Geometry check sheet. Reference: the model listing, model coordinates, mm. Face numbers are marked on the shaded views. A direction names the side the tool comes from. Give positions to 0.01 mm unless a question says otherwise; leave off trailing zeros. Loops run counter-clockwise (first coordinate to the right, second up) from the corner with the lowest first, then second, coordinate; pieces in that order, holes last. Notation, with made-up numbers: (31.25, -18.5) -> (45.25, -18.5) arc R20 cw to (45.25, -12.5) -> close; hole circle Ø4 at (37.5, 85). An arc over 180 degrees is marked (long way). One line per question, with ' | ' between items.
from build123d import *

# Parameters (mm, degrees)
SKETCH1_W      = 7.96
SKETCH1_H      = 7.96
EXTRUDE1_DEPTH = 6.3
EXTRUDE2_DEPTH = 8.96
SHELL1_T       = -1.55
EXTRUDE4_DEPTH = 4.86
SKETCH6_W      = 7.96
SKETCH6_H      = 7.96
SKETCH6_W_2    = 7.56
SKETCH6_H_2    = 7.56
EXTRUDE5_DEPTH = 0.2
FILLET1_R      = 0.05


with BuildPart() as part:
    # Sketch1 → Extrude1 (new body)
    with BuildSketch(Plane(origin=(0, 0, 0), x_dir=(1, 0, 0), z_dir=(0, 1, 0))):
        Rectangle(SKETCH1_W, SKETCH1_H)
    extrude(amount=EXTRUDE1_DEPTH)

    # Sketch2 → Extrude2 (cut, through all)
    with BuildSketch(Plane(origin=(3.98, 0, 0), x_dir=(0, 0, -1), z_dir=(1, 0, 0))):
        Polygon((-3.98, 2.2), (3.98, 6.3), (-3.98, 6.3), align=None)
    extrude(amount=-EXTRUDE2_DEPTH, mode=Mode.SUBTRACT)

    # Shell1
    shell1_openings = [part.faces().sort_by_distance(p)[0] for p in [
        (0, 0, 0),
    ]]
    offset(amount=SHELL1_T, openings=shell1_openings, kind=Kind.INTERSECTION)

    # Sketch5 → Extrude4 (cut)
    with BuildSketch(Plane(origin=(-2.43, 0, 0), x_dir=(0, 0, -1), z_dir=(1, 0, 0))):
        Polygon((-2.43, 0), (2.43, 0), (2.43, 3.915585189), (-2.43, 1.412318857), align=None)
    extrude(amount=EXTRUDE4_DEPTH, mode=Mode.SUBTRACT)

    # Sketch6 → Extrude5 (cut)
    with BuildSketch(Plane.XZ):
        Rectangle(SKETCH6_W, SKETCH6_H)
        Rectangle(SKETCH6_W_2, SKETCH6_H_2, mode=Mode.SUBTRACT)
    extrude(amount=-EXTRUDE5_DEPTH, mode=Mode.SUBTRACT)

    # Fillet1
    fillet1_edges = [part.edges().sort_by_distance(p)[0] for p in [
        (3.98, 1.2, 3.98),
        (-3.98, 1.2, 3.98),
        (0, 2.2, 3.98),
        (-3.98, 4.25, 0),
        (3.98, 4.25, 0),
        (2.43, 0.706159428, 2.43),
        (2.43, 0, 0),
        (0, 0, -2.43),
        (2.43, 1.957792594, -2.43),
        (-2.43, 1.957792594, -2.43),
        (-2.43, 0, 0),
        (-2.43, 0.706159428, 2.43),
        (0, 0, 2.43),
        (2.43, 2.663952023, 0),
        (0, 3.915585189, -2.43),
        (-2.43, 2.663952023, 0),
        (0, 1.412318857, 2.43),
        (-3.98, 0.2, 0),
        (0, 0.2, 3.98),
        (3.98, 0.2, 0),
        (0, 0.2, -3.98),
        (-3.78, 0.2, 0),
        (0, 0.2, -3.78),
        (3.78, 0.2, 0),
        (0, 0.2, 3.78),
        (-3.78, 0, 0),
        (-3.78, 0.1, 3.78),
        (0, 0, 3.78),
        (3.78, 0.1, 3.78),
        (3.78, 0, 0),
        (3.78, 0.1, -3.78),
        (0, 0, -3.78),
        (-3.78, 0.1, -3.78),
        (0, 6.3, -3.98),
        (-3.98, 3.25, -3.98),
        (3.98, 3.25, -3.98),
    ]]
    fillet(fillet1_edges, radius=FILLET1_R)


solid = part.part
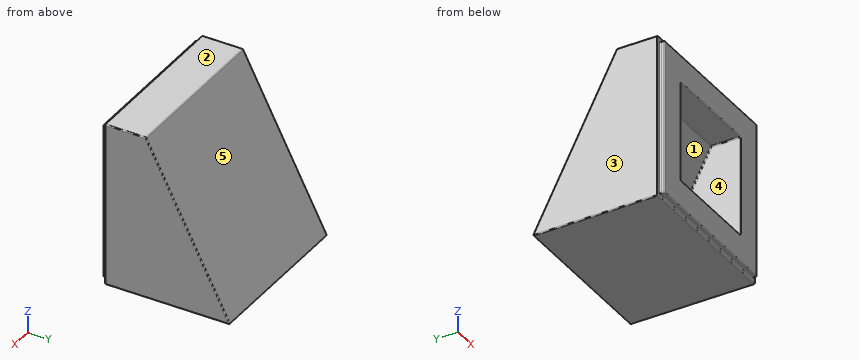
Item 1: Sectioned sample at B-B (x = -1.75). Record the cut outline in (y, z), plus the area to 3 significant figures.
Result:
outline: (0, -3.73) arc R0.05 ccw to (0.05, -3.78) -> (0.15, -3.78) arc R0.05 cw to (0.2, -3.83) -> (0.2, -3.93) arc R0.05 ccw to (0.25, -3.98) -> (6.22, -3.98) arc R0.05 ccw to (6.26, -3.91) -> (2.21, 3.95) arc R0.05 ccw to (2.17, 3.98) -> (0.25, 3.98) arc R0.05 ccw to (0.2, 3.93) -> (0.2, 3.83) arc R0.05 cw to (0.15, 3.78) -> (0.05, 3.78) arc R0.05 ccw to (0, 3.73) -> (0, 2.48) arc R0.05 ccw to (0.05, 2.43) -> (1.38, 2.43) arc R0.05 cw to (1.43, 2.4) -> (3.88, -2.36) arc R0.05 cw to (3.83, -2.43) -> (0.05, -2.43) arc R0.05 ccw to (0, -2.48) -> close | area: 20.8 mm2
Item 2: Sectioned sample at A-A (x = -3.25). Record the cut outline in (y, z), plus the area to 3 significant figures.
Result:
outline: (0, -3.73) arc R0.05 ccw to (0.05, -3.78) -> (0.15, -3.78) arc R0.05 cw to (0.2, -3.83) -> (0.2, -3.93) arc R0.05 ccw to (0.25, -3.98) -> (6.22, -3.98) arc R0.05 ccw to (6.26, -3.91) -> (2.21, 3.95) arc R0.05 ccw to (2.17, 3.98) -> (0.25, 3.98) arc R0.05 ccw to (0.2, 3.93) -> (0.2, 3.83) arc R0.05 cw to (0.15, 3.78) -> (0.05, 3.78) arc R0.05 ccw to (0, 3.73) -> close | area: 33.7 mm2
Item 3: Depth check by flat-ended pin: pin 1 Ø4 at (x, z) = (-0.5, 2) entering from +Y; pin 2 Ø2 at (x, z) = (-1.5, -2.5) entering from +Y. Enter the tip coordinate at first touch or a pass-through.
Result:
pin 1: y = 4.25 | pin 2: y = 6.05
Item 4: Scan lines: probe 1 along X at (y, z) = (0.5, 1); probe 2 along Z at (x, y) = (1, 5.5). Record each from-to range of solid material in increasing order.
Result:
probe 1: -3.98 to -2.43, 2.43 to 3.98 | probe 2: -3.98 to -2.43
Item 5: Set-up check for the marked faces 4 and 5: record each of +Z, -Z, +X, -X, +Y, -Y from which the full face is reachable in a straight line by a thin tool's end or side.
Result:
face 4: -Y | face 5: +Z, +X, -X, +Y
Item 6: Release check for a two-part mould opening along Z. For the marked faces 1, 2 and 3 record: pulls with the +Z half, pulls with the -Z half, needs draft (parallel to the pull), parting line crosses it, or undercut.
Result:
face 1: undercut | face 2: pulls with the +Z half | face 3: needs draft
